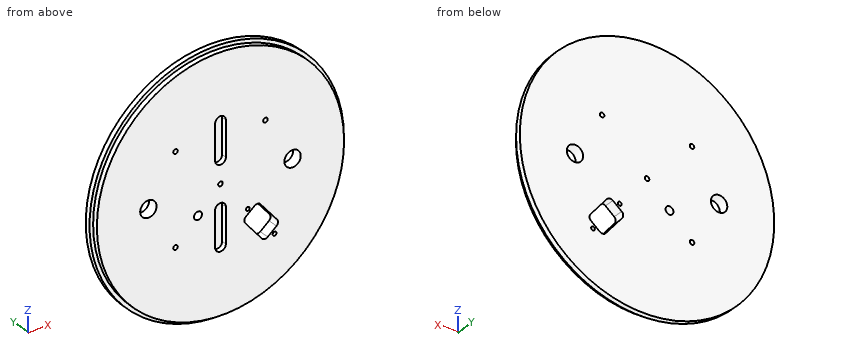
```python
from build123d import *

# Parameters (mm, degrees)
SKETCH1_R                 = 76.2
SKETCH1_R_2               = 4.9022
SKETCH1_R_3               = 1.3589
SKETCH1_R_4               = 2.38125
BOSS_EXTRUDE1_DEPTH       = 6.35
SKETCH2_R                 = 76.2
SKETCH2_R_2               = 74.041
CUT_EXTRUDE1_DEPTH        = 3.175
CUT_EXTRUDE2_START        = -3.175
CUT_EXTRUDE2_DEPTH        = 3.556
TAP_DRILL_FOR_4_40_TAP1_D = 2.2606
CUT_EXTRUDE3_DEPTH        = 7.35


with BuildPart() as part:
    # Sketch1 → Boss-Extrude1 (new body)
    with BuildSketch(Plane(origin=(0, 0, 0), x_dir=(1, 0, 0), z_dir=(0, 1, 0))):
        Circle(SKETCH1_R)
        with Locations((43.18, 0)):
            Circle(SKETCH1_R_2, mode=Mode.SUBTRACT)
        with Locations((-43.18, 0)):
            Circle(SKETCH1_R_2, mode=Mode.SUBTRACT)
        with Locations((-26.940768363, 26.940768363)):
            Circle(SKETCH1_R_3, mode=Mode.SUBTRACT)
        with Locations((26.940768363, -26.940768363)):
            Circle(SKETCH1_R_3, mode=Mode.SUBTRACT)
        with Locations((-13.470384182, 13.470384182)):
            Circle(SKETCH1_R_4, mode=Mode.SUBTRACT)
        with Locations((-26.940768363, -26.940768363)):
            Circle(SKETCH1_R_3, mode=Mode.SUBTRACT)
        Circle(SKETCH1_R_3, mode=Mode.SUBTRACT)
    extrude(amount=BOSS_EXTRUDE1_DEPTH)

    # Sketch2 → Cut-Extrude1 (cut)
    with BuildSketch(Plane.XZ):
        Circle(SKETCH2_R)
        Circle(SKETCH2_R_2, mode=Mode.SUBTRACT)
    extrude(amount=-CUT_EXTRUDE1_DEPTH, mode=Mode.SUBTRACT)

    # Sketch3 → Cut-Extrude2 (cut)
    with BuildSketch(Plane(origin=(0, 6.35, 0), x_dir=(1, 0, 0), z_dir=(0, 1, 0)).offset(CUT_EXTRUDE2_START)):
        with BuildLine():
            Line((3.2385, 34.798), (3.2385, 13.97))
            ThreePointArc((3.2385, 13.97), (0, 10.7315), (-3.2385, 13.97))
            Line((-3.2385, 13.97), (-3.2385, 34.798))
            ThreePointArc((-3.2385, 34.798), (0, 38.0365), (3.2385, 34.798))
        make_face()
        with BuildLine():
            Line((3.2385, -34.798), (3.2385, -13.97))
            ThreePointArc((3.2385, -13.97), (0, -10.7315), (-3.2385, -13.97))
            Line((-3.2385, -13.97), (-3.2385, -34.798))
            ThreePointArc((-3.2385, -34.798), (0, -38.0365), (3.2385, -34.798))
        make_face()
    extrude(amount=-CUT_EXTRUDE2_DEPTH, mode=Mode.SUBTRACT)

    # Tap Drill for #4-40 Tap1 (through all)
    with Locations(Plane(origin=(0, 6.35, 0), x_dir=(1, 0, 0), z_dir=(0, 1, 0))):
        with Locations((16.326805286, 19.457528855), (32.396495553, 38.608639962)):
            Hole(TAP_DRILL_FOR_4_40_TAP1_D / 2)

    # Sketch4 → Cut-Extrude3 (cut, through all)
    with BuildSketch(Plane(origin=(0, 6.35, 0), x_dir=(1, 0, 0), z_dir=(0, 1, 0))):
        with BuildLine():
            Line((15.169451366, 23.412825166), (20.422984157, 19.004587739))
            ThreePointArc((20.422984157, 19.004587739), (22.277040272, 18.420006091), (24.001417571, 19.317660095))
            Line((24.001417571, 19.317660095), (33.866921829, 31.074910238))
            ThreePointArc((33.866921829, 31.074910238), (34.451503477, 32.928966353), (33.553849472, 34.653343652))
            Line((33.553849472, 34.653343652), (28.300316681, 39.061581079))
            ThreePointArc((28.300316681, 39.061581079), (26.446260566, 39.646162727), (24.721883267, 38.748508722))
            Line((24.721883267, 38.748508722), (14.856379009, 26.99125858))
            ThreePointArc((14.856379009, 26.99125858), (14.271797362, 25.137202465), (15.169451366, 23.412825166))
        make_face()
    extrude(amount=-CUT_EXTRUDE3_DEPTH, mode=Mode.SUBTRACT)


solid = part.part
```
Verification items for the finished model (mm, model axes). Coordinates: 2 decimals unless noted, no trailing zeros. Write each loop counter-clockwise with the first axis right and the second up, starting at its lowest first coordinate (ties: lowest second). Pieces come first, ordered by that corner, then holes. Notation, with made-up numbers: (16, 34) - (22, 34) arc R21 ccw to (22, 41) - close; hole circle Ø5 at (18.25, 59.25). An arc over 180 degrees is marked (long way). Write item = value, one per line.
Q1. Cross-section at B-B (y = 1.25). Give the number of separate pieces and of enclosed holes in the cut face, plus the area to 3 significant figures.
Answer:
separate_pieces = 1
enclosed_holes = 12
area = 16,400 mm²
Q2. Go/stop test with flat-tipped pins: pin 1 Ø3.5 at (y, z) = (2, 29) entering from -X; pin 2 Ø2 at (x, z) = (26.94, 26.94) entering from -Y; pin 3 Ø3 at (y, z) = (5.5, 30) entering from -X; pin 4 Ø3.5 at (y, z) = (2.5, -20.5) entering from -X. Record where each tip stops, or that it passes through.
Answer:
pin_1 = -70.99
pin_2 = through
pin_3 = -70.67
pin_4 = -73.82
Q3. Cross-section at A-A (x = 43.18). Enter the section's corners in (y, z) (3 decimals), plus the area to 3 significant figures.
Answer:
outline = (0, -60.146) - (3.175, -60.146) - (3.175, -62.785) - (6.35, -62.785) - (6.35, -4.902) - (0, -4.902) - close; (0, 4.902) - (6.35, 4.902) - (6.35, 62.785) - (3.175, 62.785) - (3.175, 60.146) - (0, 60.146) - close
area = 718 mm²
Q4. Cross-section at D-D (x = -58.5). Enter the section's corners in (y, z) (3 decimals), plus the area to 3 significant figures.
Answer:
outline = (0, -45.385) - (3.175, -45.385) - (3.175, -48.828) - (6.35, -48.828) - (6.35, 48.828) - (3.175, 48.828) - (3.175, 45.385) - (0, 45.385) - close
area = 598 mm²
Q5. Cross-section at C-C (z = -48). Enter the section's corners in (x, y) (3 decimals).
Answer:
outline = (-59.181, 3.175) - (-56.374, 3.175) - (-56.374, 0) - (56.374, 0) - (56.374, 3.175) - (59.181, 3.175) - (59.181, 6.35) - (-59.181, 6.35) - close
Q6. Material ranges on L1, parallel to Z at x = 0, y = 5.25; L2, parallel to Z at x = 2.5, y = 1.75; L3, parallel to X at y = 4.5, z = -4.5, recorded low to high. Write a range as from..to.
Answer:
L1 = -76.2..-1.36, 1.36..76.2
L2 = -74..-36.86, -11.91..11.91, 36.86..74
L3 = -76.07..-45.12, -41.24..41.24, 45.12..76.07
